Autodesk Fusion 360 part; units mm, degrees
sketch "Sketch1" plane through (0, 0, 0) normal (0, 1, 0) x (1, 0, 0)
  line L0 (0, 0) -> (0, -30)
  line L1 (0, -30) -> (30, -30)
  line L2 (30, -30) -> (30, 0)
  line L3 (30, 0) -> (0, 0)
  dimension "d1" = 30
  dimension "d2" = 30
extrude "Extrude1" add sketch "Sketch1" along normal blind 8
sketch "Sketch2" plane through (0, 0, 0) normal (0, -1, 0) x (1, 0, 0)
  line L0 (0, 0) -> (30, 0)
  line L1 (30, 0) -> (30, 30)
  line L2 (30, 30) -> (0, 30)
  line L3 (0, 30) -> (0, 0)
  circle A0 centre (15, 15) radius 14
  dimension "d5" = 28
extrude "Extrude2" cut sketch "Sketch2" along normal blind 2 and the other way blind 2 contours A0
sketch "Sketch4" plane through (0, 2, 0) normal (0, -1, 0) x (1, 0, 0)
  circle A0 centre (15, 15) radius 3
  dimension "d10" = 6
extrude "Extrude3" cut sketch "Sketch4" against normal blind 6
sketch "Sketch7" plane through (0, 0, 0) normal (1, 0, 0) x (0, 1, 0)
  line L0 (8, 30) -> (8, 38)
  line L1 (8, 38) -> (-30, 38)
  line L2 (8, 30) -> (-30, 30)
  line L3 (-30, 30) -> (-30, 38)
  dimension "d40" = 8
  dimension "d41" = 38
sketch "Sketch8" plane through (0, 2, 0) normal (0, -1, 0) x (1, 0, 0)
  circle A0 centre (15, 15) radius 3
  circle A1 centre (15, 15) radius 14
sketch "Sketch10" plane through (0, 2, 0) normal (0, -1, 0) x (1, 0, 0)
  circle A0 centre (15, 4) radius 1.7
  circle A1 centre (15, 26) radius 1.7
  circle A2 centre (4, 15) radius 1.7
  circle A3 centre (26, 15) radius 1.7
  dimension "d31" = 3.4
  dimension "d32" = 3.4
  dimension "d33" = 3.4
  dimension "d34" = 3.4
extrude "Extrude5" cut sketch "Sketch10" against normal blind 6
sketch "Sketch11" plane through (0, 2, 0) normal (0, -1, 0) x (1, 0, 0)
  circle A0 centre (15, 15) radius 9
  dimension "d37" = 18
extrude "Extrude6" cut sketch "Sketch11" against normal blind 2
extrude "Extrude7" add sketch "Sketch7" along normal blind 30
sketch "Sketch14" plane through (0, 0, 30) normal (0, 0, -1) x (1, 0, 0)
  line L0 (0, 0) -> (30, 0)
  line L1 (30, 0) -> (30, 30)
  line L2 (30, 30) -> (0, 30)
  line L3 (0, 30) -> (0, 0)
  circle A0 centre (7.5, 7.5) radius 1.7
  circle A1 centre (22.5, 7.5) radius 1.7
  circle A2 centre (7.5, 22.5) radius 1.7
  circle A3 centre (22.5, 22.5) radius 1.7
  dimension "d46" = 3.4
  dimension "d47" = 3.4
  dimension "d48" = 3.4
  dimension "d49" = 3.4
extrude "Extrude8" cut sketch "Sketch14" against normal blind 8 contours A0 | A1 | A2 | A3
equation "d1 = feature1Height"
equation "d2 = mountWidth"
equation "d5 = motorDC"
equation "d10 = shaftDiameter"
equation "d31 = boltClearance"
equation "d32 = boltClearance"
equation "d33 = boltClearance"
equation "d34 = boltClearance"
equation "d40 = plateThickness"
equation "d41 = feature2Length"
equation "d46 = boltClearance"
equation "d47 = boltClearance"
equation "d48 = boltClearance"
equation "d49 = boltClearance"
equation "mountWidth = 30 mm"
equation "feature1Height = 30 mm"
equation "feature2Length = 38 mm"
equation "plateThickness = 8 mm"
equation "motorBCD = 22 mm"
equation "boltClearance = 3.4 mm"
equation "shaftDiameter = 6 mm"
equation "pilotDiameter = 18 mm"
equation "pilotDepth = 2 mm"
equation "wallHoleOffset = 7.5 mm"
equation "motorDC = 28 mm"
Work out the finished part from the listing and answer in its coordinate system (mm). A direction names the side the tool comes from. Give positions to 0.01 mm unless a question says otherwise; leave off trailing zeros. Write each loop counter-clockwise with the first axis right and the second up, starting at its lowest first coordinate (ties: lowest second). Pieces come first, ordered by that corner, then holes. Notation, with made-up numbers: (70, 10.25) - (129, 10.25) arc R16 cw to (129, 28.25) - close; hole circle Ø6 at (74.5, -28.75). An arc over 180 degrees is marked (long way). One line per item, written item: value. Start each with the question number.
1. Find section A-A (x = 15). Write down the section's boundary in (y, z).
2. For a pull along X with two mould halves and no side action, classify faces 1 (the flat face through (30, -3, 32)), 2 (the cylindrical face through (7.279, -24.186, 33.944)), 3 (the flat face through (15, -15, 30)), 4 (the flat face through (0, -3, 32)) as +X half, -X half, draft (parallel to the pull), parting line (faces both ways), or undercut.
3. Find section C-C (z = 15). Write down the section's boundary in (x, y), then the cut area to 3 significant figures.
4. Consider probe 1 along X at (y, z) = (-7, 34); probe 2 along Y at (x, z) = (22.5, 36.25); probe 3 along Y at (x, z) = (6, 36). Determine where each line is inside the solid, lowest interval first.
5. Find section B-B (y = -22.5). Write down the section's boundary in (x, z).
6. For faces 5 (the cylindrical face through (7.13, -5.84, 33.94)), 6 (the flat face through (15, 4, 11)), 7 (the flat face through (6, 0, 4)), determine the directions among +Z, -Z, +X, -X, +Y, -Y from which every point of the face is accessible in a straight line to the end or side of a thin tool.
7. Given pin 1 (4 mm diameter, centred on x = 26, z = 15, fed in from -Y); pin 2 (4 mm diameter, centred on x = 11, y = -14, fed in from -Z); pin 3 (9.5 mm diameter, centred on x = 15, z = 15, fed in from -Y), each flat-ended and moving along its own axis, determine where each tip first touches the part or whether it passes through.
8. Find section D-D (x = 3.5). Write down the section's boundary in (y, z), then the cut area to 3 significant figures.
Geometry results:
1. outline: (-30, 30) - (0, 30) - (0, 29) - (2, 29) - (2, 27.7) - (8, 27.7) - (8, 38) - (-30, 38) - close; (0, 0) - (8, 0) - (8, 2.3) - (2, 2.3) - (2, 1) - (0, 1) - close; (2, 5.7) - (8, 5.7) - (8, 12) - (4, 12) - (4, 6) - (2, 6) - close; (2, 24) - (4, 24) - (4, 18) - (8, 18) - (8, 24.3) - (2, 24.3) - close
2. face 1: +X half
2. face 2: undercut
2. face 3: draft
2. face 4: -X half
3. outline: (0, 0) - (1, 0) - (1, 2) - (2.3, 2) - (2.3, 8) - (0, 8) - close; (5.7, 2) - (6, 2) - (6, 4) - (12, 4) - (12, 8) - (5.7, 8) - close; (18, 4) - (24, 4) - (24, 2) - (24.3, 2) - (24.3, 8) - (18, 8) - close; (27.7, 2) - (29, 2) - (29, 0) - (30, 0) - (30, 8) - (27.7, 8) - close
3. area: 83.2 mm2
4. probe 1: 0 to 5.88, 9.12 to 20.88, 24.12 to 30
4. probe 2: -30 to -24.2, -20.8 to -9.2, -5.8 to 8
4. probe 3: -30 to -23.3, -21.7 to -8.3, -6.7 to 8
5. outline: (0, 30) - (5.8, 30) - (5.8, 38) - (0, 38) - close; (9.2, 30) - (20.8, 30) - (20.8, 38) - (9.2, 38) - close; (24.2, 30) - (30, 30) - (30, 38) - (24.2, 38) - close
6. face 5: +Z, -Z
6. face 6: -Y
6. face 7: -Z, +X, -X, -Y
7. pin 1: y = 2
7. pin 2: z = 30
7. pin 3: y = 4
8. outline: (-30, 30) - (0, 30) - (0, 22.98) - (2, 22.98) - (2, 16.62) - (8, 16.62) - (8, 38) - (-30, 38) - close; (0, 0) - (8, 0) - (8, 13.38) - (2, 13.38) - (2, 7.02) - (0, 7.02) - close
8. area: 493 mm2
